from build123d import *

# Parameters (mm, degrees)
SKETCH3_W                = 343
SKETCH3_H                = 5
BOSS_EXTRUDE1_DEPTH      = 35
SKETCH6_R                = 2.5
BOSS_EXTRUDE3_DEPTH      = 15
BOSS_EXTRUDE3_DEPTH_BACK = 358
BOSS_EXTRUDE4_DEPTH      = 343
SKETCH8_R                = 6
SKETCH8_R_2              = 5.999960458
CUT_EXTRUDE1_DEPTH       = 2.23071


with BuildPart() as part:
    # Sketch3 → Boss-Extrude1 (new body)
    with BuildSketch(Plane(origin=(0, 0, 0), x_dir=(1, 0, 0), z_dir=(0, 1, 0))):
        Rectangle(SKETCH3_W, SKETCH3_H)
    extrude(amount=BOSS_EXTRUDE1_DEPTH)

    # Sketch6 → Boss-Extrude3 (add, two sides)
    with BuildSketch(Plane.ZY.offset(171.5)) as boss_extrude3_sk:
        with Locations((0, 33.5)):
            Circle(SKETCH6_R)
    extrude(amount=BOSS_EXTRUDE3_DEPTH)
    extrude(boss_extrude3_sk.sketch, amount=-BOSS_EXTRUDE3_DEPTH_BACK)

    # Sketch7 → Boss-Extrude4 (add)
    with BuildSketch(Plane(origin=(171.5, 0, 0), x_dir=(0, 0, -1), z_dir=(1, 0, 0))):
        Polygon((35, -2), (42.071067812, 5.071067812), (40.656854249, 6.485281374), (34.402283019, 0.230710143), (-34.402283019, 0.230710143), (-40.656854249, 6.485281374), (-42.071067812, 5.071067812), (-35, -2), align=None)
    extrude(amount=-BOSS_EXTRUDE4_DEPTH)

    # Sketch8 → Cut-Extrude1 (cut)
    with BuildSketch(Plane(origin=(0, 0.230710143, 0), x_dir=(1, 0, 0), z_dir=(0, 1, 0))):
        with Locations((0, -24.5)):
            Circle(SKETCH8_R)
        with Locations((-49, -24.5)):
            Circle(SKETCH8_R_2)
        with Locations((-98, -24.5)):
            Circle(SKETCH8_R)
        with Locations((-147, -24.5)):
            Circle(SKETCH8_R)
        with Locations((147, -24.5)):
            Circle(SKETCH8_R)
        with Locations((98, -24.5)):
            Circle(SKETCH8_R)
        with Locations((49, -24.5)):
            Circle(SKETCH8_R_2)
        with Locations((98, 24.5)):
            Circle(SKETCH8_R)
        with Locations((147, 24.5)):
            Circle(SKETCH8_R)
        with Locations((49, 24.5)):
            Circle(SKETCH8_R_2)
        with Locations((0, 24.5)):
            Circle(SKETCH8_R)
        with Locations((-147, 24.5)):
            Circle(SKETCH8_R)
        with Locations((-98, 24.5)):
            Circle(SKETCH8_R)
        with Locations((-49, 24.5)):
            Circle(SKETCH8_R_2)
    extrude(amount=-CUT_EXTRUDE1_DEPTH, mode=Mode.SUBTRACT)


solid = part.part
Verification items for the finished model (mm, model axes). A direction names the side the tool comes from. Coordinates: 2 decimals unless noted, no trailing zeros. Loops run counter-clockwise (first coordinate to the right, second up) from the corner with the lowest first, then second, coordinate; pieces in that order, holes last. Notation, with made-up numbers: M -14.75,-13.75 L 6.25,-13.75 A27 cw 6.25,25.25 Z; hole C 71,76 d8. An arc over 180 degrees is marked long. One line per item, written item: value.
1. Section check C-C on z = -13.5. Record the cut outline in (x, y).
Answers follow:
outline: M -171.5,-2 L 171.5,-2 L 171.5,0.23 L -171.5,0.23 Z
2. Section check A-A on x = 49. Record the cut outline in (y, z), plus the area to 3 significant figures.
Answers follow:
outline: M -2,-35 L 5.07,-42.07 L 6.49,-40.66 L 0.23,-34.4 L 0.23,-30.5 L -2,-30.5 Z; M -2,-18.5 L 0.23,-18.5 L 0.23,-2.5 L 35,-2.5 L 35,-2 A2.5 ccw 35,2 L 35,2.5 L 0.23,2.5 L 0.23,18.5 L -2,18.5 Z; M -2,30.5 L 0.23,30.5 L 0.23,34.4 L 6.49,40.66 L 5.07,42.07 L -2,35 Z
area: 316 mm^2
3. Material ranges on line 1 along Z through (x, y) = (-128, 5); line 2 along Z through (x, y) = (-4, 4); line 3 along Z through (x, y) = (-117.5, 34), recorded low to high. Write a range as from..to.
Answers follow:
line 1: -42..-39.17, -2.5..2.5, 39.17..42
line 2: -41..-38.17, -2.5..2.5, 38.17..41
line 3: -2.5..2.5
4. Section check B-B on x = -136.5. Record the cut outline in (y, z).
Answers follow:
outline: M -2,-35 L 5.07,-42.07 L 6.49,-40.66 L 0.23,-34.4 L 0.23,-2.5 L 35,-2.5 L 35,-2 A2.5 ccw 35,2 L 35,2.5 L 0.23,2.5 L 0.23,34.4 L 6.49,40.66 L 5.07,42.07 L -2,35 Z
5. Section check D-D on x = 144.5. Record the cut outline in (y, z).
Answers follow:
outline: M -2,-35 L 5.07,-42.07 L 6.49,-40.66 L 0.23,-34.4 L 0.23,-29.95 L -2,-29.95 Z; M -2,-19.05 L 0.23,-19.05 L 0.23,-2.5 L 35,-2.5 L 35,-2 A2.5 ccw 35,2 L 35,2.5 L 0.23,2.5 L 0.23,19.05 L -2,19.05 Z; M -2,29.95 L 0.23,29.95 L 0.23,34.4 L 6.49,40.66 L 5.07,42.07 L -2,35 Z
6. Mould release check, pull along X, two halves, no side actions. Record for faces 3 (the cylindrical face through (-50.301, -0.869, -18.643)), 4 (the flat face through (171.5, 5, 0)), 5 (the flat face through (2.401, 3.314, 37.486)): pulls with the +X half, pulls with the -X half, needs draft (parallel to the pull), parting line crosses it, or undercut.
Answers follow:
face 3: undercut
face 4: pulls with the +X half
face 5: needs draft
7. Set-up check for faces 1 (the flat face through (2.4, 0.231, -18.7)), 2 (the flat face through (2, 2, 39)): record each of +Z, -Z, +X, -X, +Y, -Y from which the full face is reachable in a straight line by a thin tool's end or side.
Answers follow:
face 1: +X, -X, +Y
face 2: +Z, +X, -X, -Y
8. Gauge pin test, flat ends, axial feed: P1, Ø2, axis at x = -78.5, z = -8, coming from the +Y side; P2, Ø1.5, axis at x = 52, y = 9.5, coming from the +Z side; P3, Ø10.5, axis at y = 9, z = 6, coming from the -X side; P4, Ø19, axis at x = -49, z = -24.5, coming from the -Y side. Record the tip position at first contact, or that the pin passes through.
Answers follow:
P1: y = 0.23
P2: z = 2.5
P3: x = -171.5
P4: y = -2
